from build123d import *

# Parameters (mm, degrees)
CYLINDER003_R           = 7.75
CYLINDER003_DEPTH       = 24.5
CYLINDER003_PITCH_ANGLE = 90
CYLINDER002_R           = 7.75
CYLINDER002_DEPTH       = 24.5
CYLINDER002_PITCH_ANGLE = 90
CYLINDER001_R           = 7.75
CYLINDER001_DEPTH       = 24.5
CYLINDER001_PITCH_ANGLE = 90
CYLINDER_R              = 7.75
CYLINDER_DEPTH          = 24.5
CYLINDER_PITCH_ANGLE    = 90
SKETCH_W                = 70
SKETCH_H                = 90
PAD_DEPTH               = 3
SKETCH001_R             = 1.6
SKETCH001_W             = 24.556784
SKETCH001_H             = 7.470249
SKETCH001_H_2           = 7.470248
POCKET_DEPTH            = 3.001
SKETCH002_R             = 1.3
POCKET001_DEPTH         = 5
SKETCH003_W             = 20
SKETCH003_H             = 19.2
SKETCH003_W_2           = 2.2
SKETCH003_H_2           = 8.7
POCKET002_DEPTH         = 5
SKETCH004_W             = 2.5
SKETCH004_H             = 53.716673
SKETCH004_H_2           = 52.48084
PAD001_DEPTH            = 50
SKETCH005_R             = 2
POCKET003_DEPTH         = 5
SKETCH006_R             = 2
POCKET004_DEPTH         = 5


with BuildPart() as cilindro003:
    # Cylinder003 → Cylinder003 (new body)
    with BuildSketch(Plane.XY):
        Circle(CYLINDER003_R)
    extrude(amount=CYLINDER003_DEPTH)


with BuildPart() as cilindro003_1:
    # Cylinder003 pitch: moved
    add(cilindro003.part.rotate(Axis((0, 0, 0), (0, 1, 0)), CYLINDER003_PITCH_ANGLE))


with BuildPart() as cilindro003_2:
    # Cylinder003 placement: moved
    add(cilindro003_1.part.moved(Location((1, 33, -4))))


with BuildPart() as cilindro002:
    # Cylinder002 → Cylinder002 (new body)
    with BuildSketch(Plane.XY):
        Circle(CYLINDER002_R)
    extrude(amount=CYLINDER002_DEPTH)


with BuildPart() as cilindro002_1:
    # Cylinder002 pitch: moved
    add(cilindro002.part.rotate(Axis((0, 0, 0), (0, 1, 0)), CYLINDER002_PITCH_ANGLE))


with BuildPart() as cilindro002_2:
    # Cylinder002 placement: moved
    add(cilindro002_1.part.moved(Location((-26, 33, -4))))


with BuildPart() as cilindro001:
    # Cylinder001 → Cylinder001 (new body)
    with BuildSketch(Plane.XY):
        Circle(CYLINDER001_R)
    extrude(amount=CYLINDER001_DEPTH)


with BuildPart() as cilindro001_1:
    # Cylinder001 pitch: moved
    add(cilindro001.part.rotate(Axis((0, 0, 0), (0, 1, 0)), CYLINDER001_PITCH_ANGLE))


with BuildPart() as cilindro001_2:
    # Cylinder001 placement: moved
    add(cilindro001_1.part.moved(Location((1, -32, -4))))


with BuildPart() as cilindro:
    # Cylinder → Cylinder (new body)
    with BuildSketch(Plane.XY):
        Circle(CYLINDER_R)
    extrude(amount=CYLINDER_DEPTH)


with BuildPart() as cilindro_1:
    # Cylinder pitch: moved
    add(cilindro.part.rotate(Axis((0, 0, 0), (0, 1, 0)), CYLINDER_PITCH_ANGLE))


with BuildPart() as cilindro_2:
    # Cylinder placement: moved
    add(cilindro_1.part.moved(Location((-26, -32, -4))))


with BuildPart() as pocket004:
    # Sketch → Pad (new body)
    with BuildSketch(Plane.XY):
        Rectangle(SKETCH_W, SKETCH_H)
    extrude(amount=PAD_DEPTH)

    # Sketch001 → Pocket (cut, through all)
    with BuildSketch(Plane.XY.offset(3)):
        with Locations((-31, 41)):
            Circle(SKETCH001_R)
        with Locations((31, 40.99757)):
            Circle(SKETCH001_R)
        with Locations((30.962712, 23.997611)):
            Circle(SKETCH001_R)
        with Locations((-30.962712, -23.997611)):
            Circle(SKETCH001_R)
        with Locations((-31, -40.99757)):
            Circle(SKETCH001_R)
        with Locations((31, -24.002375)):
            Circle(SKETCH001_R)
        with Locations((31, -41)):
            Circle(SKETCH001_R)
        with Locations((-31, 24.002375)):
            Circle(SKETCH001_R)
        with Locations((-13.560973, 32.952)):
            Rectangle(SKETCH001_W, SKETCH001_H)
        with Locations((13.560973, 32.952)):
            Rectangle(SKETCH001_W, SKETCH001_H)
        with Locations((-13.416692, -31.992343)):
            Rectangle(SKETCH001_W, SKETCH001_H_2)
        with Locations((13.416692, -31.992343)):
            Rectangle(SKETCH001_W, SKETCH001_H_2)
    extrude(amount=-POCKET_DEPTH, mode=Mode.SUBTRACT)

    # Cut: cut Cilindro
    add(cilindro_2.part, mode=Mode.SUBTRACT)

    # Cut001: cut Cilindro001
    add(cilindro001_2.part, mode=Mode.SUBTRACT)

    # Cut002: cut Cilindro002
    add(cilindro002_2.part, mode=Mode.SUBTRACT)

    # Cut003: cut Cilindro003
    add(cilindro003_2.part, mode=Mode.SUBTRACT)


with BuildPart() as pocket004_1:
    # Cut003 placement: moved
    add(pocket004.part.moved(Location((-2, 0, -3))))

    # Sketch002 → Pocket001 (cut)
    with BuildSketch(Plane(origin=(-2, 0, 0), x_dir=(1, 0, 0), z_dir=(0, 0, 1))):
        with Locations((-14.5, 17)):
            Circle(SKETCH002_R)
        with Locations((14.5, 17)):
            Circle(SKETCH002_R)
        with Locations((-14.5, -17)):
            Circle(SKETCH002_R)
        with Locations((14.5, -17)):
            Circle(SKETCH002_R)
        with BuildLine():
            Line((-14.7, 11.879998), (-14.719215, -11.80326))
            ThreePointArc((-14.719215, -11.80326), (-13.340801, -15.147756), (-10.003866, -16.544373))
            Line((-10.003866, -16.544373), (9.305833, -16.544373))
            ThreePointArc((9.305833, -16.544373), (12.986254, -15.019893), (14.510734, -11.339472))
            Line((14.510734, 11.504763), (14.510734, -11.339472))
            ThreePointArc((14.510734, 11.504763), (13.274823, 15.056005), (9.830535, 16.564538))
            Line((-9.994001, 16.589889), (9.830535, 16.564538))
            ThreePointArc((-9.994001, 16.589889), (-13.324786, 15.211921), (-14.7, 11.879998))
        make_face()
    extrude(amount=-POCKET001_DEPTH, mode=Mode.SUBTRACT)

    # Sketch003 → Pocket002 (cut)
    with BuildSketch(Plane(origin=(-2, 0, -3), x_dir=(1, 0, 0), z_dir=(0, 0, -1))):
        with Locations((29.9, 10.5)):
            Rectangle(SKETCH003_W, SKETCH003_H)
        with Locations((26.5, -7.35)):
            Rectangle(SKETCH003_W_2, SKETCH003_H_2)
        with Locations((-26.5, 7.35)):
            Rectangle(SKETCH003_W_2, SKETCH003_H_2)
        with Locations((-29.9, -10.5)):
            Rectangle(SKETCH003_W, SKETCH003_H)
    extrude(amount=-POCKET002_DEPTH, mode=Mode.SUBTRACT)

    # Sketch004 → Pad001 (new body)
    with BuildSketch(Plane(origin=(-2, 0, 0), x_dir=(1, 0, 0), z_dir=(0, 0, 1))):
        with Locations((-18.65, -6.758337)):
            Rectangle(SKETCH004_W, SKETCH004_H)
        with Locations((18.65, 6.14042)):
            Rectangle(SKETCH004_W, SKETCH004_H_2)
    extrude(amount=PAD001_DEPTH)

    # Sketch005 → Pocket003 (cut)
    with BuildSketch(Plane(origin=(15.4, 0, -3), x_dir=(0, -1, 0), z_dir=(-1, 0, 0))):
        with Locations((-27.176525, 6.711402)):
            Circle(SKETCH005_R)
        with Locations((15.389979, 45.131245)):
            Circle(SKETCH005_R)
        with BuildLine():
            ThreePointArc((10.192183, 44.909271), (-23.272878, 44.760821), (-27.383847, 11.548891))
            Line((-27.383847, 11.548891), (-29.700115, 9.200952))
            ThreePointArc((-29.700115, 9.200952), (-30.439753, 5.326589), (-27.139361, 3.16669))
            Line((-27.139361, 3.16669), (-27.139361, 3))
            Line((-27.139361, 3), (-35.173277, 3))
            Line((-35.173277, 3), (-35.173277, 58.633105))
            Line((-1.788184, 58.633105), (-35.173277, 58.633105))
            Line((28.415094, 58.633105), (-1.788184, 58.633105))
            Line((28.415094, 24.297183), (28.415094, 58.633105))
            Line((20.052043, 24.297183), (28.415094, 24.297183))
            Line((20.038811, 25.58395), (20.052043, 24.297183))
            ThreePointArc((20.038811, 25.58395), (18.804072, 33.19525), (15.373691, 40.10097))
            Line((15.373691, 40.10097), (17.838895, 42.64968))
            ThreePointArc((17.838895, 42.64968), (17.859709, 47.592096), (12.917249, 47.589082))
            Line((10.192183, 44.909271), (12.917249, 47.589082))
        make_face()
    extrude(amount=-POCKET003_DEPTH, mode=Mode.SUBTRACT)

    # Sketch006 → Pocket004 (cut)
    with BuildSketch(Plane(origin=(-19.4, 0, -3), x_dir=(0, 1, 0), z_dir=(1, 0, 0))):
        with Locations((-27.176525, 6.711402)):
            Circle(SKETCH006_R)
        with Locations((15.389979, 45.131245)):
            Circle(SKETCH006_R)
        with BuildLine():
            ThreePointArc((10.192183, 44.909271), (-23.272878, 44.760821), (-27.383847, 11.548891))
            Line((-27.383847, 11.548891), (-29.700115, 9.200952))
            ThreePointArc((-29.700115, 9.200952), (-30.439753, 5.326589), (-27.139361, 3.16669))
            Line((-27.139361, 3.16669), (-27.139361, 3))
            Line((-27.139361, 3), (-35.173277, 3))
            Line((-35.173277, 3), (-35.173277, 58.633105))
            Line((-1.788184, 58.633105), (-35.173277, 58.633105))
            Line((28.415094, 58.633105), (-1.788184, 58.633105))
            Line((28.415094, 24.297183), (28.415094, 58.633105))
            Line((20.052043, 24.297183), (28.415094, 24.297183))
            Line((20.038811, 25.58395), (20.052043, 24.297183))
            ThreePointArc((20.038811, 25.58395), (18.804072, 33.19525), (15.373691, 40.10097))
            Line((15.373691, 40.10097), (17.838895, 42.64968))
            ThreePointArc((17.838895, 42.64968), (17.859709, 47.592096), (12.917249, 47.589082))
            Line((10.192183, 44.909271), (12.917249, 47.589082))
        make_face()
    extrude(amount=-POCKET004_DEPTH, mode=Mode.SUBTRACT)


solid = pocket004_1.part
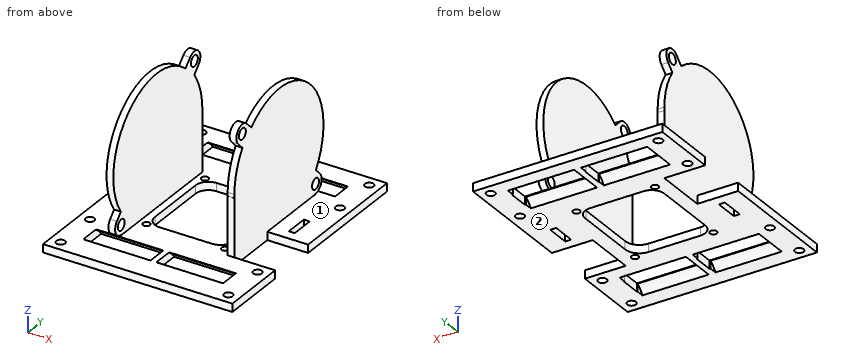
The model under review builds one solid part; all positions refer to its coordinate system, in mm. Face numbers are marked on the shaded views. Round coordinates to 2 decimals unless told otherwise and drop trailing zeros. Write each loop counter-clockwise with the first axis right and the second up, starting at its lowest first coordinate (ties: lowest second). Pieces come first, ordered by that corner, then holes. Notation, with made-up numbers: M 88,-5.75 L 126,-5.75 A16 cw 126,9.25 Z; hole C 34.25,-27.75 d1. An arc over 180 degrees is marked long. Use a Markdown table: item, result. Add a question column.
Q1. We need section B-B, the plane z = 29. State the section outline as (x, y) points.
Q2. We need section C-C, the plane x = -33. State the section outline as (y, z) points.
Q3. To check wall thickness, follow line 1 (Y direction, x = -33, z = -1.1); line 2 (X direction, y = -15, z = 25); line 3 (X direction, y = -23.5, z = 1). State the ranges of each line that lie inside material, in increasing order.
Q4. We need section A-A, the plane x = 22. State the section outline as (y, z) points.
Q5. We need section D-D, the plane y = 8. State the section outline as (x, z) points.
Q6. The part is to be moulded in two halves that separate along X. For the marked faces 1 and 2, say which applies: pulls with the +X half, pulls with the -X half, needs draft (parallel to the pull), parting line crosses it, or undercut.
Q7. Insertion check: pin 1 (1.9 mm diameter, centred on x = -33, y = -41, fed in from +Z); pin 2 (14.5 mm diameter, centred on y = 9, z = 23, fed in from -X); pin 3 (6 mm diameter, centred on x = 2.5, y = 26, fed in from +Z); pin 4 (6.5 mm diameter, centred on y = 27.18, z = 3.71, fed in from -X). Each pin has a flat end and moves straight along its axis. Give the tip position at first contact, or say it passes through.
Findings below:
| question | item | result |
|---|---|---|
| 1 | outline | M -21.9,-31.02 L -19.4,-31.02 L -19.4,19.16 L -21.9,19.16 Z; M 15.4,-19.16 L 17.9,-19.16 L 17.9,31.02 L 15.4,31.02 Z |
| 2 | outline | M -45,-3 L -42.6,-3 L -42.6,0 L -45,0 Z; M -39.4,-3 L -25.6,-3 L -25.6,0 L -39.4,0 Z; M -22.4,-3 L 0.9,-3 L 0.9,0 L -22.4,0 Z; M 20.1,-3 L 22.4,-3 L 22.4,0 L 20.1,0 Z; M 25.6,-3 L 39.4,-3 L 39.4,0 L 25.6,0 Z; M 42.6,-3 L 45,-3 L 45,0 L 42.6,0 Z |
| 3 | line 1 | y = -45 to -42.6, -39.4 to -25.6, -22.4 to 0.9, 20.1 to 22.4, 25.6 to 39.4, 42.6 to 45 |
| 3 | line 2 | x = -21.9 to -19.4, 15.4 to 17.9 |
| 3 | line 3 | x = -21.9 to -19.4 |
| 4 | outline | M -45,-3 L -38.64,-3 A7.75 cw -35.73,-0.21 L -35.73,0 L -45,0 Z; M -28.26,-0.21 A7.75 cw -25.36,-3 L -20.1,-3 L -20.1,0 L -28.26,0 Z; M -0.9,-3 L 26.36,-3 A7.75 cw 29.22,-0.24 L 29.22,0 L -0.9,0 Z; M 36.69,-0.18 A7.75 cw 39.64,-3 L 45,-3 L 45,0 L 36.69,0 Z |
| 5 | outline | M -21.9,-3 L -16.7,-3 L -16.7,0 L -19.4,0 L -19.4,43.62 L -21.9,43.62 Z; M 12.51,-3 L 23.4,-3 L 23.4,0 L 17.9,0 L 17.9,48.1 L 15.4,48.1 L 15.4,0 L 12.51,0 Z; M 25.6,-3 L 33,-3 L 33,0 L 25.6,0 Z |
| 6 | face 1 | undercut |
| 6 | face 2 | needs draft |
| 7 | pin 1 | passes through |
| 7 | pin 2 | stops at x = -21.9 |
| 7 | pin 3 | stops at z = 0 |
| 7 | pin 4 | stops at x = 15.4 |
